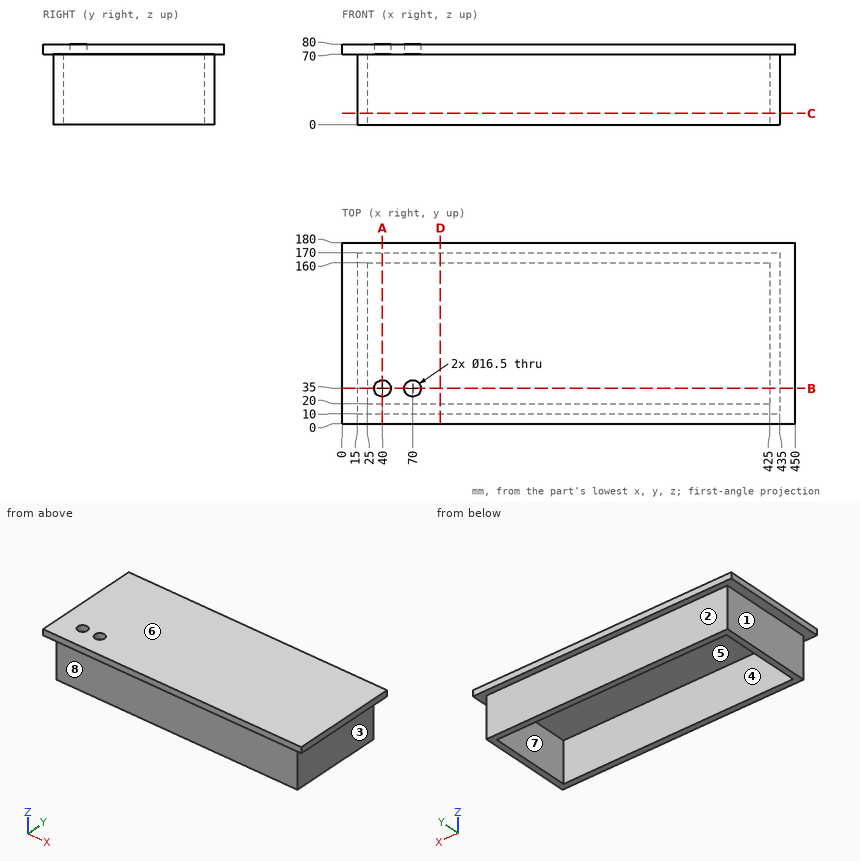
Can you work these out from the drawing? Everything is in mm from the part's minimum corner. A direction names the side the tool comes from. Give positions to 0.01 mm unless a question says otherwise; leave off trailing zeros. Order: outer loops, then holes, each group sorted by start corner. A loop starts at its lowest first (then second) coordinate and runs counter-clockwise, first axis right, second up. Notation, with made-up numbers: M -22,42.25 L 30,42.25 A23 ccw 30,68.25 Z; hole C 28.5,79 d9. An arc over 180 degrees is marked long. One line per item, written item: value.
Item 1: For pin 1 (1 mm diameter, centred on x = 255, z = 27.5, fed in from +Y); pin 2 (5 mm diameter, centred on y = 61.5, z = 63, fed in from +X); pin 3 (5 mm diameter, centred on x = 134.5, z = 16, fed in from -Y), each with a flat end and sliding along its axis, tell me the tip position at first contact or that it passes through.
Verdict:
pin 1: y = 170
pin 2: x = 435
pin 3: y = 10
Item 2: If we section it at D-D on x = 97.5: Write out the boundary of the cut face in (y, z).
Verdict:
outline: M 0,70 L 10,70 L 10,0 L 20,0 L 20,70 L 160,70 L 160,0 L 170,0 L 170,70 L 180,70 L 180,80 L 0,80 Z
Item 3: If we section it at B-B on y = 35: Write out the boundary of the cut face in (x, z).
Verdict:
outline: M 0,70 L 15,70 L 15,0 L 25,0 L 25,70 L 31.75,70 L 31.75,80 L 0,80 Z; M 48.25,70 L 61.75,70 L 61.75,80 L 48.25,80 Z; M 78.25,70 L 425,70 L 425,0 L 435,0 L 435,70 L 450,70 L 450,80 L 78.25,80 Z
Item 4: If we mould it in two halves opening along Y, with no side actions, what happens to the marked faces 5, 6, 7 and 8? For each: pulls with the +Y half, pulls with the -Y half, needs draft (parallel to the pull), parting line crosses it, or undercut.
Verdict:
face 5: undercut
face 6: needs draft
face 7: undercut
face 8: pulls with the -Y half
Item 5: Please list where these lines run through material, in increasing order: line 1 (Y direction, x = 40, z = 74.5); line 2 (X direction, y = 151.5, z = 34.5); line 3 (Y direction, x = 81, z = 40).
Verdict:
line 1: 0 to 26.75, 43.25 to 180
line 2: 15 to 25, 425 to 435
line 3: 10 to 20, 160 to 170
Item 6: For the marked faces 1, 2, 3 and 4, which set-ups out of +Z, -Z, +X, -X, +Y, -Y let a thin tool reach every point of the face, with its end or its side?
Verdict:
face 1: -Z, -X, +Y, -Y
face 2: -Z, +X, -X, +Y
face 3: -Z, +X, +Y, -Y
face 4: -Z
Item 7: If we section it at A-A on x = 40: Write out the boundary of the cut face in (y, z).
Verdict:
outline: M 0,70 L 10,70 L 10,0 L 20,0 L 20,70 L 26.75,70 L 26.75,80 L 0,80 Z; M 43.25,70 L 160,70 L 160,0 L 170,0 L 170,70 L 180,70 L 180,80 L 43.25,80 Z
Item 8: If we section it at C-C on z = 11: Write out the boundary of the cut face in (x, y).
Verdict:
outline: M 15,10 L 435,10 L 435,170 L 15,170 Z; hole M 25,20 L 425,20 L 425,160 L 25,160 Z
